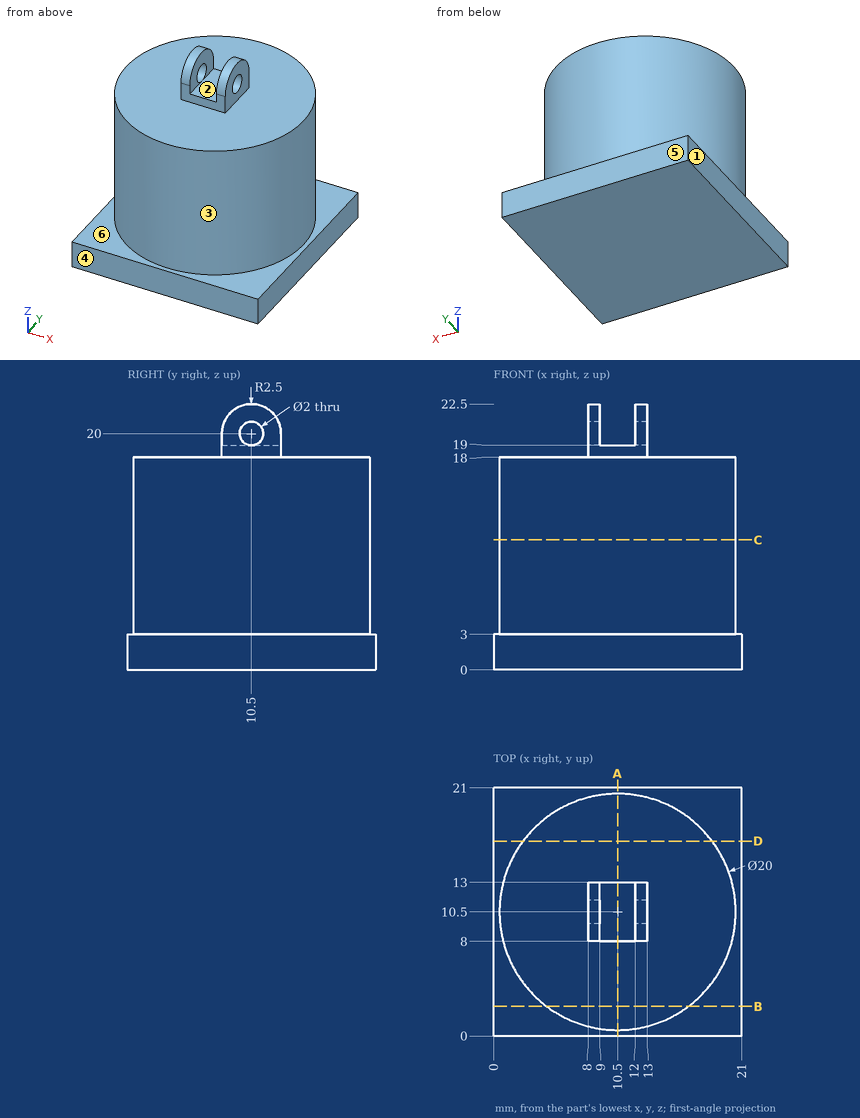
Here's the drawing with two shaded views (mm, measured from the low corner). I have some questions. A direction names the side the tool comes from. Give positions to 0.01 mm unless a question says otherwise; leave off trailing zeros. Order: outer loops, then holes, each group sorted by start corner. A loop starts at its lowest first (then second) coordinate and runs counter-clockwise, first axis right, second up. Notation, with made-up numbers: (8.5, 28.5) - (39.5, 28.5) arc R4 cw to (39.5, 34.5) - close; hole circle Ø3 at (-5, 85.5). An arc over 180 degrees is marked (long way). Use a Markdown table: item, result. Add a question column.
Q1. I'm going to push flat-ended pins straight in: pin 1 (12 mm diameter, centred on x = 11, z = 17.5, fed in from -Y); pin 2 (6 mm diameter, centred on x = 4, y = 18, fed in from +Z); pin 3 (3 mm diameter, centred on y = 10.5, z = 20, fed in from -X); pin 4 (1.3 mm diameter, centred on y = 10.5, z = 20, fed in from -X). Where does each tip first touch, or does it pass through?
Q2. If we section it at D-D on y = 16.5: Write out the boundary of the cut face in (x, z), plus the area to 3 significant figures.
Q3. Please list where these lines run through material, in increasing order: line 1 along Y through (x, z) = (12.6, 20); line 2 along Z through (x, y) = (12.75, 10.5); line 3 along X through (y, z) = (11.5, 20.75).
Q4. If we mould it in two halves opening along X, with no side actions, what happens to the marked faces 1, 2, 3 and 4? For each: released by +X, released by -X, zero draft, split by the parting line, or undercut.
Q5. If we section it at C-C on z = 11: Write out the boundary of the cut face in (x, y).
Q6. On a 3-axis mill with a long thin cutter (end or side, diameter ignored), from which of +Z, -Z, +X, -X, +Y, -Y can I reach the whole of each face in a straight line? I mean the marked faces 5 and 6. Say none if no direction works.
Q7. If we section it at A-A on x = 10.5: Write out the boundary of the cut face in (y, z), plus the area to 3 significant figures.
Q8. If we section it at B-B on y = 2.5: Write out the boundary of the cut face in (x, z), plus the area to 3 significant figures.
Answers follow:
| question | item | result |
|---|---|---|
| 1 | pin 1 | stops at y = 0.5 |
| 1 | pin 2 | stops at z = 18 |
| 1 | pin 3 | stops at x = 8 |
| 1 | pin 4 | passes through |
| 2 | outline | (0, 0) - (21, 0) - (21, 3) - (18.5, 3) - (18.5, 18) - (2.5, 18) - (2.5, 3) - (0, 3) - close |
| 2 | area | 303 mm^2 |
| 3 | line 1 | y = 8 to 9.5, 11.5 to 13 |
| 3 | line 2 | z = 0 to 19, 21 to 22.5 |
| 3 | line 3 | x = 8 to 9, 12 to 13 |
| 4 | face 1 | released by -X |
| 4 | face 2 | undercut |
| 4 | face 3 | split by the parting line |
| 4 | face 4 | zero draft |
| 5 | outline | circle Ø20 at (10.5, 10.5) |
| 6 | face 5 | +Z, -Z, +X, -X, +Y |
| 6 | face 6 | +Z |
| 7 | outline | (0, 0) - (21, 0) - (21, 3) - (20.5, 3) - (20.5, 18) - (13, 18) - (13, 19) - (8, 19) - (8, 18) - (0.5, 18) - (0.5, 3) - (0, 3) - close |
| 7 | area | 368 mm^2 |
| 8 | outline | (0, 0) - (21, 0) - (21, 3) - (16.5, 3) - (16.5, 18) - (4.5, 18) - (4.5, 3) - (0, 3) - close |
| 8 | area | 243 mm^2 |
